For this review, take the finished solid that the model builds, in its own axes (mm). Coordinates: 2 decimals unless noted, no trailing zeros. Loops run counter-clockwise (first coordinate to the right, second up) from the corner with the lowest first, then second, coordinate; pieces in that order, holes last.
1. Clearance check with a flat-ended pin moving along its axis: P1, Ø5, axis at y = 0, z = 25.4, coming from the -X side. State where the tip first meets the part, or that it passes through.
2. Take a section at B-B, the plane x = 0.7. State the section outline as (y, z) points.
3. Mouldability with a two-part tool opening along Z and no side actions: class faces 1 (the face through (0, 0, 0)), 2 (the face through (0, 19.05, 13)), 3 (the face through (0.022, 0.419, 44.445)), 4 (the face through (-0.022, 0.174, 29.365)) as pulls with the +Z half, pulls with the -Z half, needs draft (parallel to the pull), parting line crosses it, or undercut.
4. Take a section at A-A, the plane y = 0. State the section outline as (x, z) points.
5. Take a section at C-C, the plane z = 24. State the section outline as (x, y) points.
6. Take a section at D-D, the plane y = -6.5. State the section outline as (x, z) points.
7. To check wall thickness, follow probe 1 along Y at (x, z) = (0.85, 25.4); probe 2 along Y at (x, z) = (0.35, 24.5); probe 3 along Z at (x, y) = (-1, 7.5). State the ranges of each line that lie inside material, in increasing order.
```python
from build123d import *

# Parameters (mm, degrees)
SKETCH1_R           = 3.96875
BOSS_EXTRUDE1_DEPTH = 1.5875


with BuildPart() as part:
    # Sketch1 → Boss-Extrude1 (new body, symmetric)
    with BuildSketch(Plane(origin=(0, 0, 0), x_dir=(0, 0, -1), z_dir=(1, 0, 0))):
        with BuildLine():
            Line((-25.4, -19.05), (0, -19.05))
            Line((0, -19.05), (0, 19.05))
            Line((0, 19.05), (-25.4, 19.05))
            ThreePointArc((-25.4, 19.05), (-44.45, 0), (-25.4, -19.05))
        make_face()
        with Locations((-25.4, 0)):
            Circle(SKETCH1_R, mode=Mode.SUBTRACT)
    extrude(amount=BOSS_EXTRUDE1_DEPTH, both=True)


solid = part.part
```
Results list:
1. P1: passes through
2. outline: (-19.05, 0) - (19.05, 0) - (19.05, 25.4) arc R19.05 ccw to (-19.05, 25.4) - close; hole circle Ø7.94 at (0, 25.4)
3. face 1: pulls with the -Z half
3. face 2: needs draft
3. face 3: pulls with the +Z half
3. face 4: undercut
4. outline: (-1.59, 0) - (1.59, 0) - (1.59, 21.43) - (-1.59, 21.43) - close; (-1.59, 29.37) - (1.59, 29.37) - (1.59, 44.45) - (-1.59, 44.45) - close
5. outline: (-1.59, -19.05) - (1.59, -19.05) - (1.59, -3.71) - (-1.59, -3.71) - close; (-1.59, 3.71) - (1.59, 3.71) - (1.59, 19.05) - (-1.59, 19.05) - close
6. outline: (-1.59, 0) - (1.59, 0) - (1.59, 43.31) - (-1.59, 43.31) - close
7. probe 1: y = -19.05 to -3.97, 3.97 to 19.05
7. probe 2: y = -19.05 to -3.87, 3.87 to 19.05
7. probe 3: z = 0 to 42.91
